from build123d import *

# Parameters (mm, degrees)
F0_W     = 100
F0_H     = 100
F1_DEPTH = 50
F2_W     = 100
F2_H     = 100
F2_R     = 4
F3_DEPTH = 30
F4_DEPTH = 50.001
F5_R     = 5
F6_DEPTH = 100.001


with BuildPart() as f1:
    # F0 (on Top) → F1 (new body)
    with BuildSketch(Plane.XY):
        Rectangle(F0_W, F0_H)
    extrude(amount=F1_DEPTH)

    # F2 (on face) → F3 (join)
    with BuildSketch(Plane.XY.offset(50)):
        Rectangle(F2_W, F2_H)
        with Locations((-40, -40)):
            Circle(F2_R, mode=Mode.SUBTRACT)
        with Locations((40, -40)):
            Circle(F2_R, mode=Mode.SUBTRACT)
        with Locations((-40, 40)):
            Circle(F2_R, mode=Mode.SUBTRACT)
        with Locations((40, 40)):
            Circle(F2_R, mode=Mode.SUBTRACT)
    extrude(amount=F3_DEPTH)

    # F4 (cut, through all): faces of the model
    f4_faces = [f1.faces().sort_by_distance(p)[0] for p in [
        (-40, 40, 50),
        (40, 40, 50),
        (40, -40, 50),
        (-40, -40, 50),
    ]]
    extrude(f4_faces, amount=-F4_DEPTH, mode=Mode.SUBTRACT)

    # F5 (on face) → F6 (cut, through all)
    with BuildSketch(Plane(origin=(-50, 0, 0), x_dir=(0, -1, 0), z_dir=(-1, 0, 0))):
        with Locations((0, 25)):
            Circle(F5_R)
    extrude(amount=-F6_DEPTH, mode=Mode.SUBTRACT)


solid = f1.part
Here's how the part is built. I have some questions about the finished solid (model axes, mm). Give positions to 0.01 mm unless a question says otherwise; leave off trailing zeros. Order: outer loops, then holes, each group sorted by start corner. A loop starts at its lowest first (then second) coordinate and runs counter-clockwise, first axis right, second up. Notation, with made-up numbers: (74.25, 27) -> (121.25, 27) arc R23 ccw to (121.25, 52) -> close; hole circle Ø6 at (59.25, -38.75). An arc over 180 degrees is marked (long way). Use a Markdown table: item, result. Add a question column.
Item 1: Imagine slicing it at B-B on z = 25. Please give me the cut outline in (x, y).
Item 2: If we mould it in two halves opening along Y, with no side actions, what happens to faces 1 (the face through (50, -1, 39)), 2 (the face through (-1, 50, 39)), 3 (the face through (-0.7, 1.08, 20.12))? For each: pulls with the +Y half, pulls with the -Y half, needs draft (parallel to the pull), parting line crosses it, or undercut.
Item 3: Imagine slicing it at D-D on z = 6. Please give me the cut outline in (x, y), plus the area to 3 significant figures.
Item 4: Imagine slicing it at A-A on x = -40. Please give me the cut outline in (y, z).
Item 5: Will these pins go through, and if not, where does the flat tip stop? pin 1 (10.5 mm diameter, centred on x = 40, y = -40, fed in from +Z); pin 2 (8 mm diameter, centred on y = 0, z = 25, fed in from -X).
Item 6: Imagine slicing it at C-C on y = 0. Please give me the cut outline in (x, z).
Item 7: I need wall thicknesses on line 1 (Y direction, x = 40, z = 13); line 2 (Y direction, x = -40, z = 22); line 3 (Z direction, x = 6, y = 0). Which ranges of each line are inside material? Lowest first, please.
Data:
| question | item | result |
|---|---|---|
| 1 | outline | (-50, -50) -> (50, -50) -> (50, -5) -> (-50, -5) -> close; (-50, 5) -> (50, 5) -> (50, 50) -> (-50, 50) -> close; hole circle Ø8 at (-40, -40); hole circle Ø8 at (-40, 40); hole circle Ø8 at (40, -40); hole circle Ø8 at (40, 40) |
| 2 | face 1 | needs draft |
| 2 | face 2 | pulls with the +Y half |
| 2 | face 3 | undercut |
| 3 | outline | (-50, -50) -> (50, -50) -> (50, 50) -> (-50, 50) -> close; hole circle Ø8 at (-40, -40); hole circle Ø8 at (-40, 40); hole circle Ø8 at (40, -40); hole circle Ø8 at (40, 40) |
| 3 | area | 9,800 mm² |
| 4 | outline | (-50, 0) -> (-44, 0) -> (-44, 80) -> (-50, 80) -> close; (-36, 0) -> (36, 0) -> (36, 80) -> (-36, 80) -> close; (44, 0) -> (50, 0) -> (50, 80) -> (44, 80) -> close; hole circle Ø10 at (0, 25) |
| 5 | pin 1 | stops at z = 80 |
| 5 | pin 2 | passes through |
| 6 | outline | (-50, 0) -> (50, 0) -> (50, 20) -> (-50, 20) -> close; (-50, 30) -> (50, 30) -> (50, 80) -> (-50, 80) -> close |
| 7 | line 1 | y = -50 to -44, -36 to 36, 44 to 50 |
| 7 | line 2 | y = -50 to -44, -36 to -4, 4 to 36, 44 to 50 |
| 7 | line 3 | z = 0 to 20, 30 to 80 |
